Verification items for this drawing (mm, ordinates from the low corner). A direction names the side the tool comes from. Coordinates: 2 decimals unless noted, no trailing zeros. Order: outer loops, then holes, each group sorted by start corner. A loop starts at its lowest first (then second) coordinate and runs counter-clockwise, first axis right, second up.
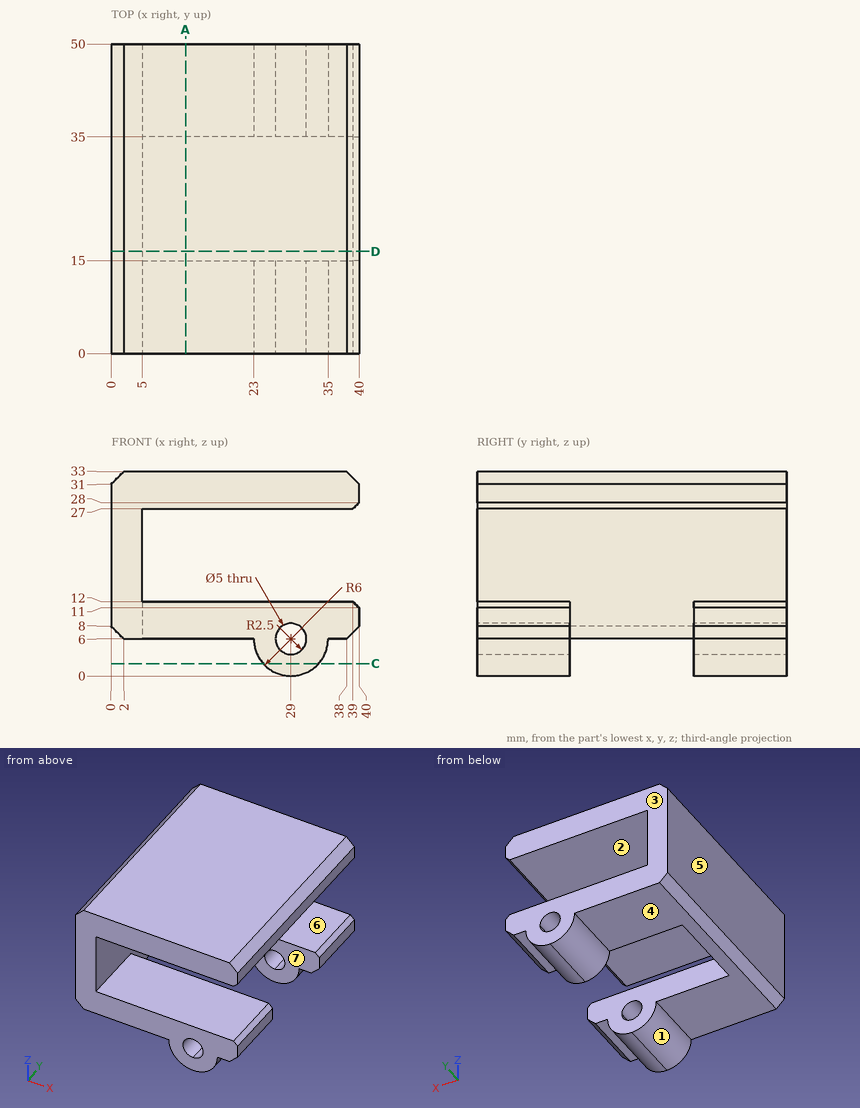
(1) Thickness scan on probe 1 along Z at (x, y) = (29, 11); probe 2 along Z at (x, y) = (15, 8); probe 3 along Y at (x, z) = (19.5, 11). Record the ranges inside material, lowest first.
Filled in:
probe 1: z = 0 to 3.5, 8.5 to 12, 27 to 33
probe 2: z = 6 to 12, 27 to 33
probe 3: y = 0 to 15, 35 to 50
(2) Cross-section at C-C (z = 2). Enter the section's corners in (x, y).
Filled in:
outline: (24.53, 0) - (33.47, 0) - (33.47, 15) - (24.53, 15) - close; (24.53, 35) - (33.47, 35) - (33.47, 50) - (24.53, 50) - close
(3) Go/stop test with flat-tipped pins: P1, Ø23, axis at x = 11.5, y = 18.5, coming from the -Z side; P2, Ø6, axis at y = 13, z = 4.5, coming from the +X side; P3, Ø1.5, axis at x = 14.5, z = 13.5, coming from the -Y side; P4, Ø10.5, axis at y = 22.5, z = 13.5, coming from the +X side. Record where each tip stops, or that it passes through.
Filled in:
P1: stops at z = 6
P2: stops at x = 39.5
P3: passes through
P4: stops at x = 5
(4) Tool access check on the marked faces 4, 5, 6 and 7. Record the directions out of +Z, -Z, +X, -X, +Y, -Y that give a thin tool (end or side, any length) a straight path to the whole face; none if there is none.
Filled in:
face 4: -Z, -X, +Y, -Y
face 5: +Z, -Z, -X, +Y, -Y
face 6: +X, +Y, -Y
face 7: -Z, +X
(5) Release check for a two-part mould opening along Z. For the marked faces 1, 2 and 3 record: +Z half, -Z half, draft (parallel to the pull), parting line (faces both ways), or undercut.
Filled in:
face 1: -Z half
face 2: undercut
face 3: draft
(6) Cross-section at D-D (y = 16.5). Enter the section's corners in (x, z).
Filled in:
outline: (0, 8) - (2, 6) - (5, 6) - (5, 27) - (39, 27) - (40, 28) - (40, 31) - (38, 33) - (2, 33) - (0, 31) - close
(7) Cross-section at A-A (x = 12). Enter the section's corners in (y, z).
Filled in:
outline: (0, 6) - (15, 6) - (15, 12) - (0, 12) - close; (0, 27) - (50, 27) - (50, 33) - (0, 33) - close; (35, 6) - (50, 6) - (50, 12) - (35, 12) - close
